Autodesk Inventor part; units mm, degrees
ref_plane "YZ Plane" through (0, 0, 0) normal (1, 0, 0) x (0, 1, 0)
ref_plane "XZ Plane" through (0, 0, 0) normal (0, 1, 0) x (-1, 0, 0)
ref_plane "XY Plane" through (0, 0, 0) normal (0, 0, 1) x (1, 0, 0)
sketch "Sketch3" plane through (0, 0, 0) normal (0, 1, 0) x (-1, 0, 0)
  circle A0 centre (0, 0) radius 17.75
  dimension "d32" = 35.5
extrude "Extrusion4" add sketch "Sketch3" along normal blind 12.7
sketch "Sketch4" plane through (0, 12.7, 0) normal (0, 1, 0) x (1, 0, 0)
  circle A0 centre (0, 0) radius 17.75
  circle A1 centre (0, 0) radius 17.75
  circle A2 centre (0, 0) radius 17.75
  circle A3 centre (0, 0) radius 17.65
  dimension "d35" = 0.1
extrude "Extrusion5" add sketch "Sketch4" along normal blind 1
fillet "Fillet1" radius 1 1 edges at (-17.65, 12.7, 0)
equation "\"d32\" = iciclesPlugD"
equation "\"d33\" = chairThickness"
equation "\"moduleHeight\" = 96"
equation "\"moduleMountD\" = 6.8"
equation "\"moduleCornerR\" = 5"
equation "\"d4\" = moduleCornerR"
equation "\"d5\" = moduleMountD"
equation "\"d6\" = moduleMountD"
equation "\"d8\" = moduleMountD"
equation "\"d10\" = moduleMountD"
equation "\"moduleOpeningR\" = 25"
equation "\"d13\" = moduleOpeningR"
equation "\"thickness\" = 6"
equation "\"d15\" = thickness"
equation "\"d16\" = 0"
equation "\"iciclesMountD\" = 42.5"
equation "\"d17\" = iciclesMountD"
equation "\"clearanceM3\" = 3.6"
equation "\"d18\" = clearanceM3"
equation "\"d21\" = 360deg"
equation "\"d0\" = moduleHeight"
equation "\"iciclesBaseOuterD\" = 48"
equation "\"iciclesPlugD\" = 35.5"
equation "\"chairThickness\" = 12.7"
equation "\"isiclesBaseThickness\" = 3"
properties part number "Module_bottom_Icicles26_v2_3DPrint"
Read the model definition and answer for the solid it produces. Units are mm, in the model's axes. Coordinates: 2 decimals unless noted, no trailing zeros. Order: outer loops, then holes, each group sorted by start corner. A loop starts at its lowest first (then second) coordinate and runs counter-clockwise, first axis right, second up. Notation, with made-up numbers: (-9, -15) - (22, -15) arc R20 cw to (22, -8) - close; hole circle Ø9 at (-17, 13). An arc over 180 degrees is marked (long way). Answer as a JSON object with one key per item and string values. Group by question number.
Item 1: Flat-ended cylindrical pins translate along their axes: P1, Ø3, axis at x = 14, z = -6, coming from the +Y side; P2, Ø2, axis at x = -3, y = 2.5, coming from the +Z side; P3, Ø21, axis at x = 0, z = 0, coming from the -Y side; P4, Ø3, axis at x = -3.5, y = 12, coming from the -Z side. Find the tip coordinate at first contact, or state that the pin passes through.
Item 2: Section A-A (y = 11.5) is taken. Give the vertices of the cut face in (x, z), plus the area to 3 significant figures.
Item 3: The mould has two halves that part along X. Classify faces 1 (the face through (0, 12.7, 0)), 2 (the face through (0, 0, 0)): +X half, -X half, draft (parallel to the pull), parting line (faces both ways), or undercut.
Item 4: Consider probe 1 along Y at (x, z) = (0, 2); probe 2 along Z at (x, y) = (0.5, 8); probe 3 along Z at (x, y) = (-8, 6.5). Determine where each line is inside the solid, lowest interval first. Write a range as from..to.
Results are:
{
 "1": {"P1": "stops at y = 12.7", "P2": "stops at z = 17.64", "P3": "stops at y = 0", "P4": "stops at z = -17.64"},
 "2": {"outline": "circle Ø35.5 at (0, 0)", "area": "990 mm^2"},
 "3": {"face 1": "undercut", "face 2": "draft"},
 "4": {"probe 1": "y = 0..12.7", "probe 2": "z = -17.74..17.74", "probe 3": "z = -15.84..15.84"}
}
